Could you check a few things on this model? Use its own coordinates, in mm. Face numbers are marked on the shaded views. A direction names the side the tool comes from. Coordinates: 2 decimals unless noted, no trailing zeros. Loops run counter-clockwise (first coordinate to the right, second up) from the corner with the lowest first, then second, coordinate; pieces in that order, holes last. Notation, with made-up numbers: (-29, 36) -> (-9, 36) arc R26 cw to (-9, 53) -> close; hole circle Ø1 at (-7, 6.25). An arc over 180 degrees is marked (long way). One line per question, with ' | ' between items. Start each with the question number.
(1) Suppose I cut it at C-C (y = 16). Please give me the cut outline in (x, z), plus the area to 3 significant figures.
(2) If I drill on line 1 along Z through (x, y) = (-20, 12); line 2 along Y through (x, z) = (-35.5, -31); line 3 along X through (y, z) = (7.5, 21.5), over which ranges is the centre line in solid material (lowest first)?
(3) Which directions (+Z, -Z, +X, -X, +Y, -Y) give clear straight access to the entire face, cutting with the end or side of a thin tool? Please do the marked faces 1, 2, 3 and 4.
(4) Suppose I cut it at D-D (z = -49.5). Please give me the cut outline in (x, y), plus the area to 3 significant figures.
(5) I'm going to push flat-ended pins straight in: pin 1 Ø5 at (x, y) = (-31, 11) entering from +Z; pin 2 Ø3 at (y, z) = (13.5, 20) entering from -X; pin 3 Ø8.5 at (x, y) = (-31.5, 10) entering from -Z; pin 4 Ø10 at (y, z) = (8.5, -37.5) entering from -X. Where does each tip first touch, or does it pass through?
(6) Suppose I cut it at A-A (x = -32.5). Please give me the cut outline in (y, z) (1 decimal).
(7) Suppose I cut it at B-B (z = 25). Please give me the cut outline in (x, y).
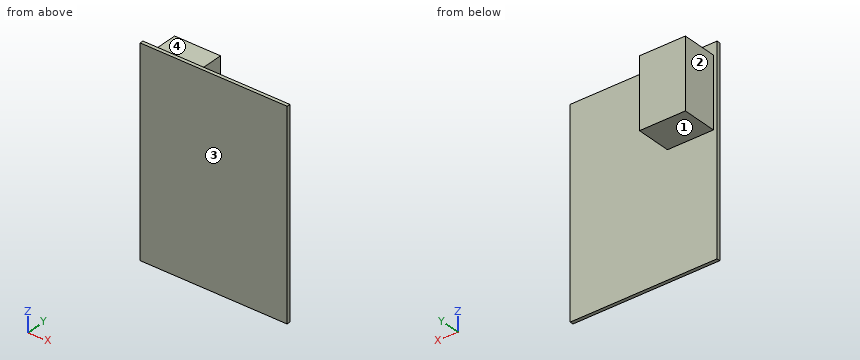
Autodesk Inventor part; units mm, degrees
ref_plane "YZ Plane" through (0, 0, 0) normal (1, 0, 0) x (0, 1, 0)
ref_plane "XZ Plane" through (0, 0, 0) normal (0, 1, 0) x (-1, 0, 0)
ref_plane "XY Plane" through (0, 0, 0) normal (0, 0, 1) x (1, 0, 0)
sketch "Sketch1" plane through (0, 0, 0) normal (0, 1, 0) x (-1, 0, 0)
  line L0 (39.8244, 42.085) -> (-31.1756, 42.085)
  line L1 (-31.1756, 42.085) -> (-31.1756, -55.915)
  line L2 (-31.1756, -55.915) -> (39.8244, -55.915)
  line L3 (39.8244, -55.915) -> (39.8244, 42.085)
  point P0 (0, 0)
  dimension "d0" = 71
  dimension "d1" = 98
extrude "Extrusion1" add sketch "Sketch1" along normal blind 1.66
sketch "Sketch2" plane through (0, 1.66, 0) normal (0, 1, 0) x (1, 0, 0)
  line L0 (-38.0351, -2.7975) -> (-15.8351, -2.7975)
  line L1 (-15.8351, -2.7975) -> (-15.8351, -36.4975)
  line L2 (-15.8351, -36.4975) -> (-38.0351, -36.4975)
  line L3 (-38.0351, -36.4975) -> (-38.0351, -2.7975)
  point P0 (0, 0)
  dimension "d4" = 33.7
  dimension "d5" = 22.2
extrude "Extrusion2" add sketch "Sketch2" along normal blind 17
sketch "Sketch3" plane through (0, 1.66, 0) normal (0, 1, 0) x (1, 0, 0)
  point P0 (0, 0)
properties part number "Board"
Checks:
1) outline: (-38.04, 2.8) -> (-15.84, 2.8) -> (-15.84, 36.5) -> (-38.04, 36.5) -> close | area: 748 mm^2
2) line 1: z = 2.8 to 36.5 | line 2: y = 0 to 1.66 | line 3: x = -38.04 to -15.84
3) face 1: -Z, +X, -X, +Y | face 2: +Z, -Z, -X, +Y | face 3: +Z, -Z, +X, -X, -Y | face 4: +Z, +X, -X, +Y
4) outline: (-39.82, 0) -> (31.18, 0) -> (31.18, 1.66) -> (-39.82, 1.66) -> close | area: 118 mm^2
5) pin 1: stops at z = 36.5 | pin 2: stops at x = -38.04 | pin 3: stops at z = 2.8 | pin 4: passes through
6) outline: (0, -55.9) -> (1.7, -55.9) -> (1.7, 2.8) -> (18.7, 2.8) -> (18.7, 36.5) -> (1.7, 36.5) -> (1.7, 42.1) -> (0, 42.1) -> close
7) outline: (-39.82, 0) -> (31.18, 0) -> (31.18, 1.66) -> (-15.84, 1.66) -> (-15.84, 18.66) -> (-38.04, 18.66) -> (-38.04, 1.66) -> (-39.82, 1.66) -> close
